```python
from build123d import *

# Parameters (mm, degrees)
F0_W     = 30
F0_H     = 12
F0_R     = 3
F0_R_2   = 3.4
F1_DEPTH = 20
F2_D     = 6.8
F2_DEPTH = 23.75
F2_TIP   = 2.0429261047
F3_SIZE  = 0.5


with BuildPart() as f1:
    # F0 (on Front) → F1 (new body)
    with BuildSketch(Plane.XZ):
        Rectangle(F0_W, F0_H)
        with Locations((-10, 0)):
            Circle(F0_R, mode=Mode.SUBTRACT)
        Circle(F0_R_2, mode=Mode.SUBTRACT)
        with Locations((10, 0)):
            Circle(F0_R, mode=Mode.SUBTRACT)
        Circle(F0_R_2)
    extrude(amount=F1_DEPTH)

    # F2
    with Locations(Plane(origin=(0, 0, 0), x_dir=(1, 0, 0), z_dir=(0, 1, 0))):
        with Locations((0, 0)):
            Hole(F2_D / 2, depth=F2_DEPTH)
            with Locations((0, 0, -(F2_DEPTH + F2_TIP / 2))):  # 118° drill point
                Cone(0, F2_D / 2, F2_TIP, mode=Mode.SUBTRACT)

    # F3
    f3_edges = [f1.edges().sort_by_distance(p)[0] for p in [
        (15, -10, 6),
        (-15, -10, 6),
        (0, 0, 6),
        (0, -20, 6),
        (-15, -10, -6),
        (15, -10, -6),
        (0, 0, -6),
        (0, -20, -6),
        (-15, 0, 0),
        (-15, -20, 0),
        (15, 0, 0),
        (15, -20, 0),
        (-7, -10, 0),
        (-13, 0, 0),
        (-13, -20, 0),
        (-3.4, 0, 0),
        (3.4, -10, 0),
        (-3.4, -20, 0),
        (13, -10, 0),
        (7, 0, 0),
        (7, -20, 0),
    ]]
    chamfer(f3_edges, length=F3_SIZE)


solid = f1.part
```
Here's how the part is built. I have some questions about the finished solid (model axes, mm). Round coordinates to 2 decimals unless told otherwise and drop trailing zeros. Order: outer loops, then holes, each group sorted by start corner. A loop starts at its lowest first (then second) coordinate and runs counter-clockwise, first axis right, second up. Notation, with made-up numbers: M 21.5,-22.5 L 44.5,-22.5 A19 cw 44.5,-12.5 Z; hole C -16,39.5 d1. An arc over 180 degrees is marked long. Use CSV: the item, a comma, the result in double quotes.
1) If we mould it in two halves opening along Z, with no side actions, what happens to faces 1 (the cylindrical face through (0.74, -10.13, 3.32)), 2 (the flat face through (3, -20, 3)), 3 (the flat face through (0, -10, 6))? For each: pulls with the +Z half, pulls with the -Z half, needs draft (parallel to the pull), parting line crosses it, or undercut.
Taken from the geometry:
face 1,"undercut"
face 2,"needs draft"
face 3,"pulls with the +Z half"
2) I want a section at C-C (y = -7.25). List the corners of the cut face in (x, z) for me.
Taken from the geometry:
outline,"M -15,-5.5 L -14.5,-6 L 14.5,-6 L 15,-5.5 L 15,5.5 L 14.5,6 L -14.5,6 L -15,5.5 Z; hole C -10,0 d6; hole C 0,0 d6.8; hole C 10,0 d6"
3) I want a section at A-A (x = 0). List the corners of the cut face in (y, z) for me.
Taken from the geometry:
outline,"M -20,-5.5 L -19.5,-6 L -0.5,-6 L 0,-5.5 L 0,-3.9 L -0.5,-3.4 L -19.5,-3.4 L -20,-3.9 Z; M -20,3.9 L -19.5,3.4 L -0.5,3.4 L 0,3.9 L 0,5.5 L -0.5,6 L -19.5,6 L -20,5.5 Z"
4) I'm going to push a flat-ended pin straight in: P1, Ø5.5, axis at x = 10, z = 0, coming from the +Y side. Where does the tip first touch, or does it pass through?
Taken from the geometry:
P1,"through"
5) I need wall thicknesses on line 1 along Z through (x, y) = (10, -6.5); line 2 along X through (y, z) = (-11.5, 2); line 3 along X through (y, z) = (-16.75, 0.5). Which ranges of each line are inside material? Lowest first, please. Write a range as [from, to].
Taken from the geometry:
line 1,"[-6, -3], [3, 6]"
line 2,"[-15, -12.24], [-7.76, -2.75], [2.75, 7.76], [12.24, 15]"
line 3,"[-15, -12.96], [-7.04, -3.36], [3.36, 7.04], [12.96, 15]"
6) I want a section at B-B (z = 0). Count the separate pieces of the cut face and the enclosed holes in it, then the cut area to 3 significant figures.
Taken from the geometry:
separate pieces,"4"
enclosed holes,"0"
area,"222 mm^2"
7) I want a section at D-D (x = 10). List the corners of the cut face in (y, z) for me.
Taken from the geometry:
outline,"M -20,-5.5 L -19.5,-6 L -0.5,-6 L 0,-5.5 L 0,-3.5 L -0.5,-3 L -19.5,-3 L -20,-3.5 Z; M -20,3.5 L -19.5,3 L -0.5,3 L 0,3.5 L 0,5.5 L -0.5,6 L -19.5,6 L -20,5.5 Z"
